Verification items for the finished model (mm, model axes). Give positions to 0.01 mm unless a question says otherwise; leave off trailing zeros. Order: outer loops, then holes, each group sorted by start corner. A loop starts at its lowest first (then second) coordinate and runs counter-clockwise, first axis right, second up. Notation, with made-up numbers: (-21, -20.75) -> (-12, -20.75) arc R12 cw to (-12, 1.25) -> close; hole circle Ø7 at (21.25, -5). An arc over 180 degrees is marked (long way). Return JSON: item names as keys, results as strings. Group by question number.
(1) Cross-section at B-B on y = 1.85. Enter the section's corners in (x, z) (3 decimals), then the cut area to 3 significant figures.
(2) Cross-section at C-C on x = -16. Enter the section's corners in (y, z), then the cut area to 3 significant figures.
(3) Cross-section at D-D on z = 26. Enter the section's corners in (x, y), then the cut area to 3 significant figures.
(4) Cross-section at A-A on z = 38. Enter the section's corners in (x, y).
(5) Thickness scan on line 1 along Z through (x, y) = (6, 4.1); line 2 along X through (y, z) = (4.35, 46.5); line 3 along Z through (x, y) = (-1, 4.05). Record the ranges inside material, lowest first.
from build123d import *

# Parameters (mm, degrees)
BOSS_EXTRUDE1_DEPTH = 4.7625


with BuildPart() as part:
    # Sketch1 → Boss-Extrude1 (new body)
    with BuildSketch(Plane(origin=(0, 0, 0), x_dir=(1, 0, 0), z_dir=(0, 1, 0))):
        with BuildLine():
            Line((22.994624733, -31.524992416), (-18.204730368, -55.415445829))
            ThreePointArc((-18.204730368, -55.415445829), (-24.10202239, -52.817624121), (-24.351569793, -46.378334027))
            Line((-24.351569793, -46.378334027), (35.179941753, 3.113165809))
            Line((35.179941753, 3.113165809), (81.92289285, -10.7327271))
            Line((81.92289285, -10.7327271), (71.73313232, -45.132782137))
            Line((71.73313232, -45.132782137), (24.990181224, -31.286889228))
            ThreePointArc((24.990181224, -31.286889228), (23.967852385, -31.200180886), (22.994624733, -31.524992416))
        make_face()
    extrude(amount=BOSS_EXTRUDE1_DEPTH)


solid = part.part
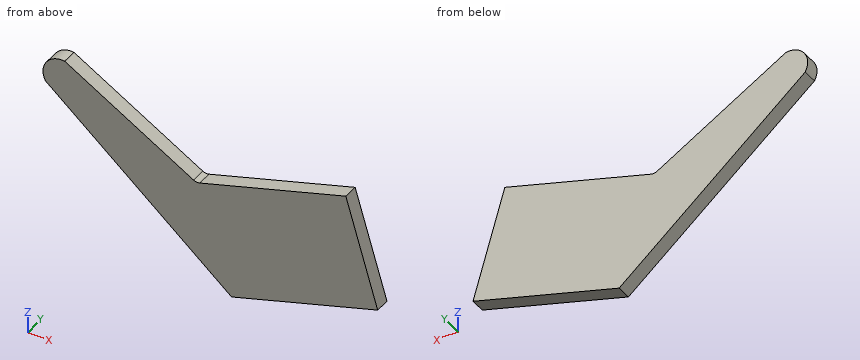
Verdict:
{
 "1": {"outline": "(-24.352, 46.378) -> (35.18, -3.113) -> (81.923, 10.733) -> (71.733, 45.133) -> (24.99, 31.287) arc R2.54 cw to (22.995, 31.525) -> (-18.205, 55.415) arc R6.08 ccw to start", "area": "2,800 mm²"},
 "2": {"outline": "(0, 39.44) -> (4.76, 39.44) -> (4.76, 54.14) -> (0, 54.14) -> close", "area": "70.0 mm²"},
 "3": {"outline": "(0.16, 0) -> (77.4, 0) -> (77.4, 4.76) -> (0.16, 4.76) -> close", "area": "368 mm²"},
 "4": {"outline": "(-14.27, 0) -> (11.83, 0) -> (11.83, 4.76) -> (-14.27, 4.76) -> close; (47.65, 0) -> (73.85, 0) -> (73.85, 4.76) -> (47.65, 4.76) -> close"},
 "5": {"line 1": "21.15 to 41.38", "line 2": "-24.42 to -2.83", "line 3": "26.97 to 45.44"}
}
